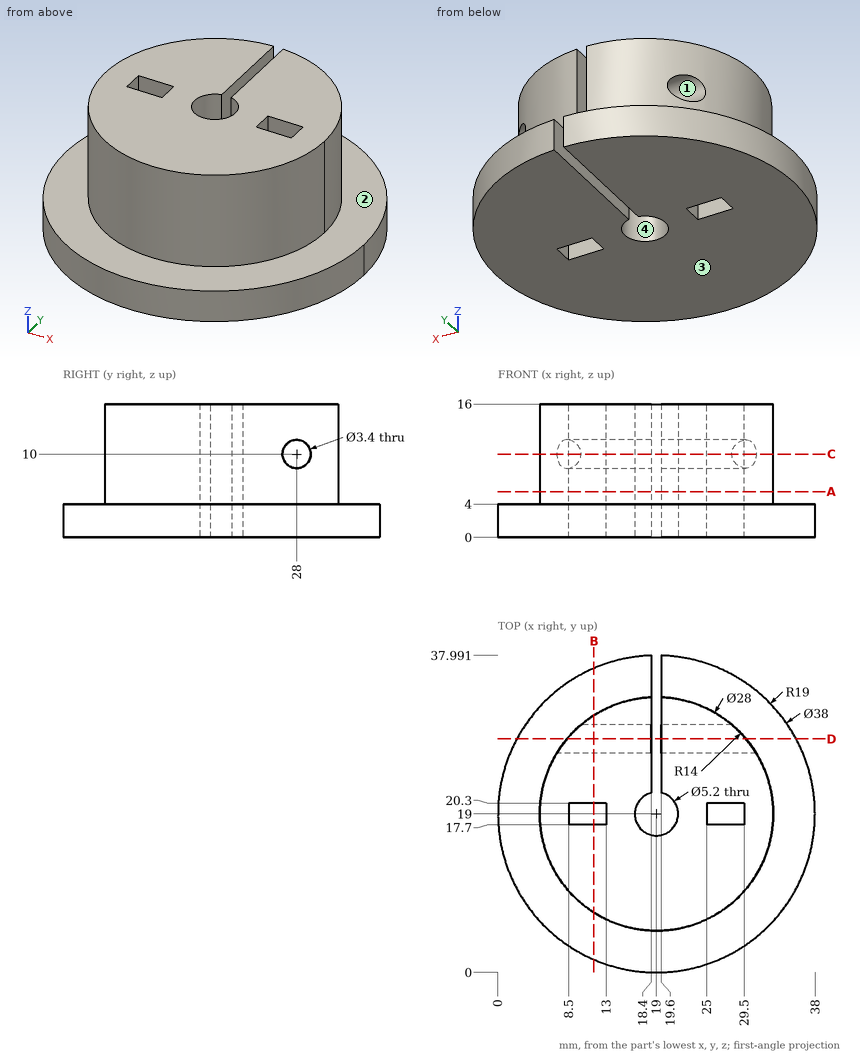
Drawing for the job (mm, zero at the part's lowest x, y, z). A direction names the side the tool comes from. Give positions to 0.01 mm unless a question says otherwise; leave off trailing zeros. Loops run counter-clockwise (first coordinate to the right, second up) from the corner with the lowest first, then second, coordinate; pieces in that order, holes last.
Item 1: Which spindle directions (+Z, -Z, +X, -X, +Y, -Y) get a long thin tool onto all of the face, cutting with end or side? Do the marked faces 1 and 2. Say none if no direction does.
Check values:
face 1: +X, -X
face 2: +Z
Item 2: Slice it at D-D (y = 28). Write the cut outline in (x, z), plus the area to 3 significant figures.
Check values:
outline: (2.27, 0) - (18.4, 0) - (18.4, 8.3) - (8.28, 8.3) - (8.28, 4) - (2.27, 4) - close; (8.28, 11.7) - (18.4, 11.7) - (18.4, 16) - (8.28, 16) - close; (19.6, 0) - (35.73, 0) - (35.73, 4) - (29.72, 4) - (29.72, 8.3) - (19.6, 8.3) - close; (19.6, 11.7) - (29.72, 11.7) - (29.72, 16) - (19.6, 16) - close
area: 303 mm2
Item 3: Slice it at B-B (x = 11.5). Write the cut outline in (y, z).
Check values:
outline: (1.54, 0) - (17.7, 0) - (17.7, 16) - (7.18, 16) - (7.18, 4) - (1.54, 4) - close; (20.3, 0) - (36.46, 0) - (36.46, 4) - (30.82, 4) - (30.82, 16) - (20.3, 16) - close; hole circle Ø3.4 at (28, 10)
Item 4: Drop flat-ended pins along their axis: P1, Ø5.5, axis at y = 28, z = 10, coming from the -X side; P2, Ø3, axis at x = 15.5, z = 5, coming from the -Y side; P3, Ø3, axis at y = 19.5, z = 11.5, coming from the -X side; P4, Ø2, axis at y = 28, z = 10, coming from the -X side. Give the stop position or say it passes through.
Check values:
P1: stops at x = 6.47
P2: stops at y = 0.15
P3: stops at x = 5
P4: passes through
Item 5: Mould opens along Y. For the marked faces 3 and 4 say: +Y half, -Y half, draft (parallel to the pull), parting line (faces both ways), or undercut.
Check values:
face 3: draft
face 4: undercut
Item 6: Slice it at A-A (z = 5.5). Write the cut outline in (x, y).
Check values:
outline: (18.4, 21.53) - (18.4, 32.99) arc R14 ccw (long way) to (19.6, 32.99) - (19.6, 21.53) arc R2.6 cw (long way) to start; hole (8.5, 17.7) - (13, 17.7) - (13, 20.3) - (8.5, 20.3) - close; hole (25, 17.7) - (29.5, 17.7) - (29.5, 20.3) - (25, 20.3) - close
Item 7: Drill centre lines: line 1 along X through (y, z) = (19, 3.75); line 2 along Z through (x, y) = (12, 28); line 3 along X through (y, z) = (20, 11) (1 decimal). Where is each one in solid material? Low to high.
Check values:
line 1: x = 0 to 8.5, 13 to 16.4, 21.6 to 25, 29.5 to 38
line 2: z = 0 to 8.3, 11.7 to 16
line 3: x = 5 to 8.5, 13 to 16.6, 21.4 to 25, 29.5 to 33
Item 8: Slice it at C-C (z = 10). Write the cut outline in (x, y), plus the area to 3 significant figures.
Check values:
outline: (7.05, 26.3) arc R14 ccw (long way) to (30.95, 26.3) - (19.6, 26.3) - (19.6, 21.53) arc R2.6 cw (long way) to (18.4, 21.53) - (18.4, 26.3) - close; (9.97, 29.7) - (18.4, 29.7) - (18.4, 32.99) arc R14 ccw to start; (19.6, 29.7) - (28.03, 29.7) arc R14 ccw to (19.6, 32.99) - close; hole (8.5, 17.7) - (13, 17.7) - (13, 20.3) - (8.5, 20.3) - close; hole (25, 17.7) - (29.5, 17.7) - (29.5, 20.3) - (25, 20.3) - close
area: 489 mm2
